Source: CAD feature listing. Evaluate the final solid. Frame: model axes, mm. Face numbers are marked on the shaded views. A direction names the side the tool comes from. Give positions to 0.01 mm unless a question says otherwise; leave off trailing zeros. Loops run counter-clockwise (first coordinate to the right, second up) from the corner with the lowest first, then second, coordinate; pieces in that order, holes last.
Autodesk Inventor part; units mm, degrees
ref_plane "YZ Plane" through (0, 0, 0) normal (1, 0, 0) x (0, 1, 0)
ref_plane "XZ Plane" through (0, 0, 0) normal (0, 1, 0) x (-1, 0, 0)
ref_plane "XY Plane" through (0, 0, 0) normal (0, 0, 1) x (1, 0, 0)
sketch "Sketch1" plane through (0, 0, 0) normal (0, 0, 1) x (1, 0, 0)
  circle A0 centre (0, 0) radius 3
  dimension "d0" = 6
extrude "Extrusion1" add sketch "Sketch1" along normal blind 6
sketch "Sketch2" plane through (0, 0, 0) normal (0, 0, 1) x (1, 0, 0)
  circle A0 centre (0, 0) radius 4.9 construction
  line L0 (2.829, 4.9) -> (-2.829, 4.9)
  line L1 (0, -6.86) -> (0, 6.86)
  line L2 (-2.829, 4.9) -> (-5.658, 0)
  line L3 (-5.658, 0) -> (-2.829, -4.9)
  line L4 (-2.829, -4.9) -> (2.829, -4.9)
  line L5 (2.829, -4.9) -> (5.658, 0)
  line L6 (5.658, 0) -> (2.829, 4.9)
  point P0 (0, 4.9)
  point P1 (-4.2435, 2.45)
  point P2 (-4.2435, -2.45)
  point P3 (0, -4.9)
  point P4 (4.2435, -2.45)
  point P5 (4.2435, 2.45)
  point P6 (-5.658, 0)
  point P7 (5.658, 0)
  dimension "d3" = 9.8
  dimension "d6" = 360
extrude "Extrusion2" add sketch "Sketch2" against normal blind 5
thread "Thread1"
properties part number "Screw"
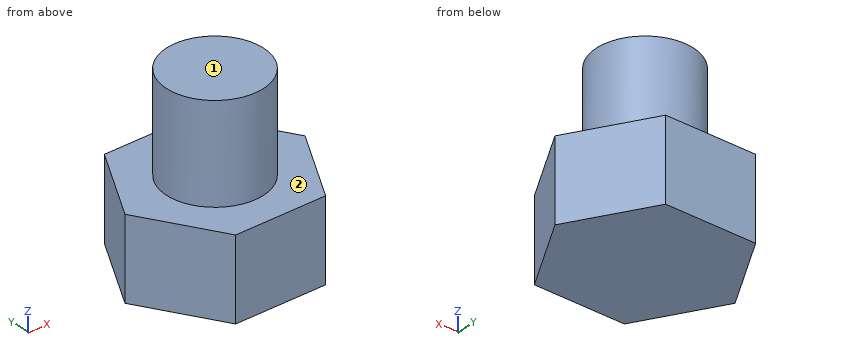
(1) Reachability of the marked faces 1 and 2 from +Z, -Z, +X, -X, +Y, -Y: full face, straight path, thin tool, end or side. Return the list, or none.
A:
face 1: +Z, +X, -X, +Y, -Y
face 2: +Z
(2) First-contact query: pin 1 (1 mm diameter, centred on y = -4, z = 3.5, fed in from +X); pin 2 (1.5 mm diameter, centred on y = -1.5, z = 1, fed in from +X); pin 3 (4 mm diameter, centred on y = 2, z = 1.5, fed in from +X); pin 4 (4 mm diameter, centred on x = -4, z = -2, fed in from +Y). Flat tips, straight axial feed; report the tip coordinate or a pass-through.
A:
pin 1: passes through
pin 2: stops at x = 2.9
pin 3: stops at x = 5.27
pin 4: stops at y = 4.9
(3) Section D-D, the plane z = 0.5. Return the cut outline in (x, y), then the cut area to 3 significant figures.
A:
outline: circle Ø6 at (0, 0)
area: 28.3 mm2
(4) Section A-A, the plane x = 0. Return the cut outline in (y, z).
A:
outline: (-4.9, -5) - (4.9, -5) - (4.9, 0) - (3, 0) - (3, 6) - (-3, 6) - (-3, 0) - (-4.9, 0) - close
(5) Ray query, line 1 along Z through (x, y) = (0, 3.25); line 2 along Y through (x, z) = (2.5, 1.25); line 3 along X through (y, z) = (4.75, -2.75). Return the intervals inside material, ascending.
A:
line 1: z = -5 to 0
line 2: y = -1.66 to 1.66
line 3: x = -2.92 to 2.92
(6) Section B-B, the plane z = -1.75. Return the cut outline in (x, y), then the cut area to 3 significant figures.
A:
outline: (-5.66, 0) - (-2.83, -4.9) - (2.83, -4.9) - (5.66, 0) - (2.83, 4.9) - (-2.83, 4.9) - close
area: 83.2 mm2
(7) Section C-C, the plane y = 0.75. Return the cut outline in (x, z), then the cut area to 3 significant figures.
A:
outline: (-5.22, -5) - (5.22, -5) - (5.22, 0) - (2.9, 0) - (2.9, 6) - (-2.9, 6) - (-2.9, 0) - (-5.22, 0) - close
area: 87.1 mm2
